Input: dimensioned drawing with shaded views. Units: mm. Origin: part minimum x, y, z. Give positions to 0.01 mm unless a question says otherwise; leave off trailing zeros. Write each loop counter-clockwise with the first axis right and the second up, starting at its lowest first coordinate (ties: lowest second). Pieces come first, ordered by that corner, then holes. Notation, with made-up numbers: (41, 34) - (81, 34) arc R7 cw to (81, 43) - close; hole circle Ø2 at (25.5, 78). An arc over 180 degrees is marked (long way). Answer as a JSON object with one key per item and string values. Group by question number.
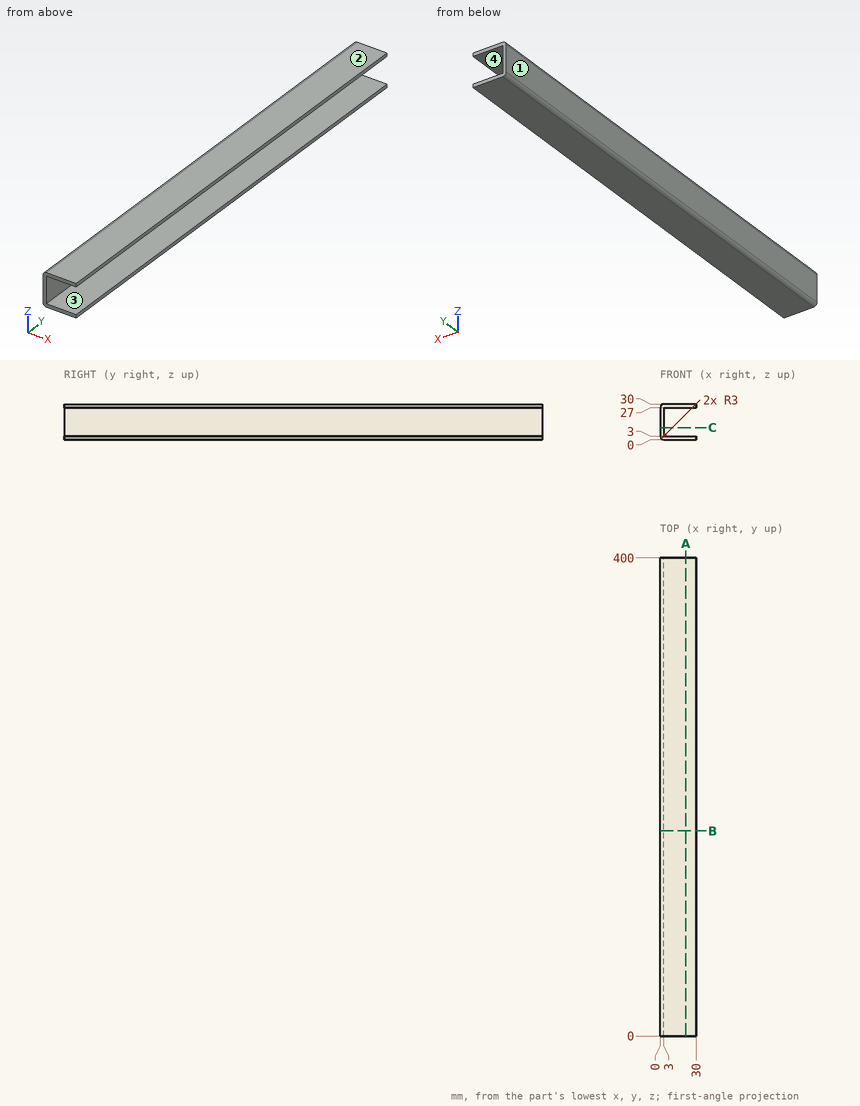
1) Line query: line 1 along Z through (x, y) = (24.75, 141); line 2 along X through (y, z) = (256, 26.25); line 3 along X through (y, z) = (253.5, 2.75). Output: solid intervals per line, ascending. Write a range as from..to.
2) Cut plane C-C on z = 10.25. Return the cut outline in (x, y).
3) Cut plane A-A on x = 21.5. Return the cut outline in (y, z), and give its area (3 significant figures).
4) Pin query (flat end, axial travel): P1, Ø2, axis at y = 310.5, z = 7.5, coming from the -X side; P2, Ø1.5, axis at y = 175, z = 14.5, coming from the +X side. Return the tip coordinate at first contact, or that it passes through.
5) Mould query, pull axis Z, two halves, no side actions, for the marked faces 1, 2, 3 and 4. Classes: +Z half, -Z half, draft (parallel to the pull), parting line (faces both ways), or undercut.
6) Cut plane B-B on y = 171.5. Return the cut outline in (x, z).
Filled in:
{
 "1": {"line 1": "z = 0..3, 27..30", "line 2": "x = 0..3", "line 3": "x = 0.01..30"},
 "2": {"outline": "(0, 0) - (3, 0) - (3, 400) - (0, 400) - close"},
 "3": {"outline": "(0, 0) - (400, 0) - (400, 3) - (0, 3) - close; (0, 27) - (400, 27) - (400, 30) - (0, 30) - close", "area": "2,400 mm²"},
 "4": {"P1": "stops at x = 0", "P2": "stops at x = 3"},
 "5": {"face 1": "draft", "face 2": "+Z half", "face 3": "undercut", "face 4": "undercut"},
 "6": {"outline": "(0, 3) arc R3 ccw to (3, 0) - (30, 0) - (30, 3) - (3, 3) - (3, 27) - (30, 27) - (30, 30) - (3, 30) arc R3 ccw to (0, 27) - close"}
}
